The figure shows three views and two pictorial views of one solid part (mm, origin at its lowest corner). Answer the questions. A direction names the side the tool comes from. Round coordinates to 2 decimals unless told otherwise and drop trailing zeros. Order: outer loops, then holes, each group sorted by start corner. A loop starts at its lowest first (then second) coordinate and runs counter-clockwise, first axis right, second up. Notation, with made-up numbers: (10.25, 21) - (50.25, 21) arc R21 cw to (50.25, 60) - close; hole circle Ø2 at (-13.5, 63.25). An arc over 180 degrees is marked (long way). Write item = value, one per line.
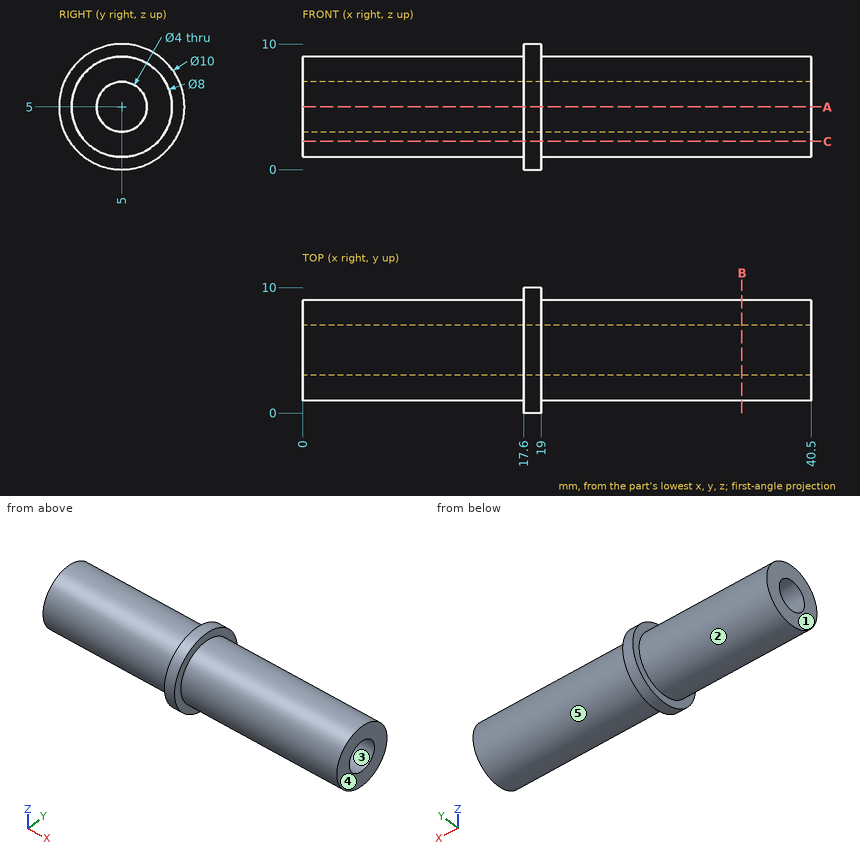
Q1. Determine the mould class of the marked faces 3, 4 and 5 for opening direction Y: released by +Y, released by -Y, zero draft, split by the parting line, or undercut.
Model answer:
face_3 = undercut
face_4 = zero draft
face_5 = split by the parting line
Q2. Section A-A on z = 5 is taken. Determine the outline of the cut face in (x, y), then the cut area to 3 significant figures.
Model answer:
outline = (0, 1) - (17.6, 1) - (17.6, 0) - (19, 0) - (19, 1) - (40.5, 1) - (40.5, 3) - (0, 3) - close; (0, 7) - (40.5, 7) - (40.5, 9) - (19, 9) - (19, 10) - (17.6, 10) - (17.6, 9) - (0, 9) - close
area = 165 mm^2
Q3. Flat-ended cylindrical pins translate along their axes: P1, Ø1.5, axis at x = 12, z = 4, coming from the +Y side; P2, Ø1, axis at x = 12.5, y = 1.5, coming from the -Z side; P3, Ø1.5, axis at x = 35.5, z = 1.5, coming from the +Y side. Find the tip coordinate at first contact, or state that the pin passes through.
Model answer:
P1 = 8.99
P2 = 2.35
P3 = 7.9
Q4. For the marked faces 1 and 2, determine the directions among +Z, -Z, +X, -X, +Y, -Y from which every point of the face is accessible in a straight line to the end or side of a thin tool.
Model answer:
face_1 = +Z, -Z, -X, +Y, -Y
face_2 = -X
Q5. Find the intervals of material crossed by line 1 (Z direction, x = 8.5, y = 5); line 2 (Z direction, x = 16.5, y = 5.5), in increasing order. Write a range as from..to.
Model answer:
line_1 = 1..3, 7..9
line_2 = 1.03..3.06, 6.94..8.97
Q6. Section B-B on x = 35 is taken. Determine the outline of the cut face in (y, z).
Model answer:
outline = circle Ø8 at (5, 5); hole circle Ø4 at (5, 5)
Q7. Section C-C on z = 2.25 is taken. Determine the outline of the cut face in (x, y), then the cut area to 3 significant figures.
Model answer:
outline = (0, 2.1) - (17.6, 2.1) - (17.6, 0.82) - (19, 0.82) - (19, 2.1) - (40.5, 2.1) - (40.5, 7.9) - (19, 7.9) - (19, 9.18) - (17.6, 9.18) - (17.6, 7.9) - (0, 7.9) - close
area = 239 mm^2
